```python
from build123d import *

# Parameters (mm, degrees)
CROQUIS1_W                      = 64
CROQUIS1_H                      = 120
CROQUIS1_R                      = 1.5
CROQUIS1_W_2                    = 2
CROQUIS1_H_2                    = 40
SALIENTE_EXTRUIR1_DEPTH         = 1
PLIEGUE_START                   = 63.746512
PLIEGUE_CROQUIZADO1_OUTLINE_W   = 120
PLIEGUE_CROQUIZADO1_OUTLINE_H   = 1
PLIEGUE_CROQUIZADO1_DEPTH       = 9.933488
PLIEGUE_START_2                 = 62.786512
PLIEGUE_CROQUIZADO1_2_OUTLINE_R = 1.5
PLIEGUE_CROQUIZADO1_2_DEPTH     = 1.213488
PLIEGUE_START_3                 = -121
PLIEGUE_CROQUIZADO1_3_DEPTH     = 122
PLIEGUE_START_4                 = -120
PLIEGUE_CROQUIZADO1_4_DEPTH     = 120
CORTAR_EXTRUIR1_REACH           = 138.485
CORTAR_EXTRUIR2_DEPTH           = 184
REDONDEO1_R                     = 4


with BuildPart() as part:
    # Croquis1 → Saliente-Extruir1 (new body)
    # profile 1 of 5: a face of its own
    with BuildSketch(Plane(origin=(0, 0, 0), x_dir=(0, 1, 0), z_dir=(0, 0, 1))):
        with Locations((32, 60)):
            Rectangle(CROQUIS1_W, CROQUIS1_H)
    # profile 2 of 5: a face of its own
    with BuildSketch(Plane(origin=(0, 0, 0), x_dir=(0, 1, 0), z_dir=(0, 0, 1))):
        Polygon((64, 120), (64, 0), (67.68, 0), (67.68, 25), (67.68, 40), (67.68, 80), (67.68, 95), (67.68, 120), align=None)
    # profile 3 of 5: a face of its own
    with BuildSketch(Plane(origin=(0, 0, 0), x_dir=(0, 1, 0), z_dir=(0, 0, 1))):
        Polygon((67.68, 40), (67.68, 25), (73.68, 25), (73.68, 40), (69.68, 40), align=None)
        with Locations(Location((69.68, 30, 0), (0, 0, 270))):
            Circle(CROQUIS1_R, mode=Mode.SUBTRACT)
    # profile 4 of 5: a face of its own
    with BuildSketch(Plane(origin=(0, 0, 0), x_dir=(0, 1, 0), z_dir=(0, 0, 1))):
        Polygon((73.68, 95), (67.68, 95), (67.68, 80), (69.68, 80), (73.68, 80), align=None)
        with Locations(Location((69.68, 90, 0), (0, 0, 270))):
            Circle(CROQUIS1_R, mode=Mode.SUBTRACT)
    # profile 5 of 5: a face of its own
    with BuildSketch(Plane(origin=(0, 0, 0), x_dir=(0, 1, 0), z_dir=(0, 0, 1))):
        with Locations((68.68, 60)):
            Rectangle(CROQUIS1_W_2, CROQUIS1_H_2)
    extrude(amount=SALIENTE_EXTRUIR1_DEPTH)

    # Pliegue croquizado1: read off the stored shape, not the designer's step
    # Pliegue croquizado1 outline → Pliegue croquizado1 (cut)
    with BuildSketch(Plane(origin=(0, 0, 0), x_dir=(1, 0, 0), z_dir=(0, 1, 0)).offset(PLIEGUE_START)):
        with Locations((-60, -0.5)):
            Rectangle(PLIEGUE_CROQUIZADO1_OUTLINE_W, PLIEGUE_CROQUIZADO1_OUTLINE_H)
    extrude(amount=PLIEGUE_CROQUIZADO1_DEPTH, mode=Mode.SUBTRACT)

    # Pliegue croquizado1 2 outline → Pliegue croquizado1 2 (add)
    with BuildSketch(Plane(origin=(0, 0, 0), x_dir=(1, 0, 0), z_dir=(0, 1, 0)).offset(PLIEGUE_START_2)):
        Polygon((-95, -11.495486979), (-80, -11.495486979), (-80, -7.495486979), (-40, -7.495486979), (-40, -11.495486979), (-25, -11.495486979), (-25, -5.495486979), (0, -5.495486979), (0, -1), (-120, -1), (-120, -5.495486979), (-95, -5.495486979), align=None)
        with Locations((-90, -7.495486979)):
            Circle(PLIEGUE_CROQUIZADO1_2_OUTLINE_R, mode=Mode.SUBTRACT)
        with Locations((-30, -7.495486979)):
            Circle(PLIEGUE_CROQUIZADO1_2_OUTLINE_R, mode=Mode.SUBTRACT)
    extrude(amount=PLIEGUE_CROQUIZADO1_2_DEPTH)

    # Pliegue croquizado1 3 outline → Pliegue croquizado1 3 (cut)
    with BuildSketch(Plane.YZ.offset(PLIEGUE_START_3)):
        with BuildLine():
            Line((63, 11.495486979), (62.786512, 11.495486979))
            Line((62.786512, 11.495486979), (62.786512, 1.656905608))
            ThreePointArc((62.786512, 1.656905608), (62.945569917, 2.013423228), (63, 2.4))
            Line((63, 2.4), (63, 11.495486979))
        make_face()
        with BuildLine():
            Line((64, 1), (64, 2.4))
            ThreePointArc((64, 2.4), (63.297056275, 0.702943725), (61.6, 0))
            Line((61.6, 0), (63.746512, 0))
            Line((63.746512, 0), (63.746512, 1))
            Line((63.746512, 1), (64, 1))
        make_face()
    extrude(amount=PLIEGUE_CROQUIZADO1_3_DEPTH, mode=Mode.SUBTRACT)

    # Pliegue croquizado1 4 outline → Pliegue croquizado1 4 (add)
    with BuildSketch(Plane.YZ.offset(PLIEGUE_START_4)):
        with BuildLine():
            Line((62.786512, 1), (62.786512, 1.656905608))
            ThreePointArc((62.786512, 1.656905608), (62.278110556, 1.175187331), (61.6, 1))
            Line((61.6, 1), (62.786512, 1))
        make_face()
    extrude(amount=PLIEGUE_CROQUIZADO1_4_DEPTH)

    # Simetría1: part across plane


with BuildPart() as part_1:
    add(part.part)
    add(part.part.mirror(Plane(origin=(0, 0, 1), x_dir=(0, 0, 1), z_dir=(0, 1, 0))))

    # Croquis7 → Cortar-Extruir1 (cut, up to next)
    with BuildSketch(Plane(origin=(0, 0, 0), x_dir=(-1, 0, 0), z_dir=(0, 0, -1)), mode=Mode.PRIVATE) as cortar_extruir1_sk1:
        with BuildLine():
            Line((35, 45.000000776), (35, -45.000000776))
            ThreePointArc((35, -45.000000776), (40.000000388, -50), (45, -45))
            Line((45, -45), (45, 45))
            ThreePointArc((45, 45), (40.000000388, 50), (35, 45.000000776))
        make_face()
    cortar_extruir1_tool1 = extrude(cortar_extruir1_sk1.sketch, amount=-CORTAR_EXTRUIR1_REACH, mode=Mode.PRIVATE) & part_1.part
    # Croquis7 → Cortar-Extruir1 (cut, up to next)
    with BuildSketch(Plane(origin=(0, 0, 0), x_dir=(-1, 0, 0), z_dir=(0, 0, -1)), mode=Mode.PRIVATE) as cortar_extruir1_sk2:
        with BuildLine():
            Line((15, 45.000000776), (15, -45.000000776))
            ThreePointArc((15, -45.000000776), (20.000000388, -50), (25, -45))
            Line((25, -45), (25, 45))
            ThreePointArc((25, 45), (20.000000388, 50), (15, 45.000000776))
        make_face()
    cortar_extruir1_tool2 = extrude(cortar_extruir1_sk2.sketch, amount=-CORTAR_EXTRUIR1_REACH, mode=Mode.PRIVATE) & part_1.part
    # Croquis7 → Cortar-Extruir1 (cut, up to next)
    with BuildSketch(Plane(origin=(0, 0, 0), x_dir=(-1, 0, 0), z_dir=(0, 0, -1)), mode=Mode.PRIVATE) as cortar_extruir1_sk3:
        with BuildLine():
            Line((55, 45.000000776), (55, -45.000000776))
            ThreePointArc((55, -45.000000776), (60.000000388, -50), (65, -45))
            Line((65, -45), (65, 45))
            ThreePointArc((65, 45), (60.000000388, 50), (55, 45.000000776))
        make_face()
    cortar_extruir1_tool3 = extrude(cortar_extruir1_sk3.sketch, amount=-CORTAR_EXTRUIR1_REACH, mode=Mode.PRIVATE) & part_1.part
    # Croquis7 → Cortar-Extruir1 (cut, up to next)
    with BuildSketch(Plane(origin=(0, 0, 0), x_dir=(-1, 0, 0), z_dir=(0, 0, -1)), mode=Mode.PRIVATE) as cortar_extruir1_sk4:
        with BuildLine():
            Line((75, 45.000000776), (75, -45.000000776))
            ThreePointArc((75, -45.000000776), (80.000000388, -50), (85, -45))
            Line((85, -45), (85, 45))
            ThreePointArc((85, 45), (80.000000388, 50), (75, 45.000000776))
        make_face()
    cortar_extruir1_tool4 = extrude(cortar_extruir1_sk4.sketch, amount=-CORTAR_EXTRUIR1_REACH, mode=Mode.PRIVATE) & part_1.part
    # Croquis7 → Cortar-Extruir1 (cut, up to next)
    with BuildSketch(Plane(origin=(0, 0, 0), x_dir=(-1, 0, 0), z_dir=(0, 0, -1)), mode=Mode.PRIVATE) as cortar_extruir1_sk5:
        with BuildLine():
            Line((95, 45.000000776), (95, -45.000000776))
            ThreePointArc((95, -45.000000776), (100.000000388, -50), (105, -45))
            Line((105, -45), (105, 45))
            ThreePointArc((105, 45), (100.000000388, 50), (95, 45.000000776))
        make_face()
    cortar_extruir1_tool5 = extrude(cortar_extruir1_sk5.sketch, amount=-CORTAR_EXTRUIR1_REACH, mode=Mode.PRIVATE) & part_1.part
    add(cortar_extruir1_tool1.solids().sort_by_distance((-40, 0, 0))[0], mode=Mode.SUBTRACT)
    add(cortar_extruir1_tool2.solids().sort_by_distance((-20, 0, 0))[0], mode=Mode.SUBTRACT)
    add(cortar_extruir1_tool3.solids().sort_by_distance((-60, 0, 0))[0], mode=Mode.SUBTRACT)
    add(cortar_extruir1_tool4.solids().sort_by_distance((-80, 0, 0))[0], mode=Mode.SUBTRACT)
    add(cortar_extruir1_tool5.solids().sort_by_distance((-100, 0, 0))[0], mode=Mode.SUBTRACT)

    # Croquis8 → Cortar-Extruir2 (cut)
    with BuildSketch(Plane.XZ.offset(64)):
        Polygon((-80, 11.495486979), (-85, 11.495486979), (-85, 5.495486979), (-80, 5.495486979), (-40, 5.495486979), (-35, 5.495486979), (-35, 11.495486979), (-40, 11.495486979), (-40, 7.495486979), (-80, 7.495486979), align=None)
    extrude(amount=-CORTAR_EXTRUIR2_DEPTH, mode=Mode.SUBTRACT)

    # Redondeo1
    redondeo1_edges = [part_1.edges().sort_by_distance(p)[0] for p in [
        (-95, -63.5, 11.495486979),
        (-25, -63.5, 11.495486979),
        (-25, 63.5, 11.495486979),
        (-95, 63.5, 11.495486979),
        (-35, 63.5, 11.495486979),
        (-85, 63.5, 11.495486979),
        (-35, -63.5, 11.495486979),
        (-85, -63.5, 11.495486979),
    ]]
    fillet(redondeo1_edges, radius=REDONDEO1_R)


solid = part_1.part
```
Geometry check sheet. Reference: the model listing, model coordinates, mm. A direction names the side the tool comes from. Coordinates: 2 decimals unless noted, no trailing zeros. Loops run counter-clockwise (first coordinate to the right, second up) from the corner with the lowest first, then second, coordinate; pieces in that order, holes last. Notation, with made-up numbers: (81, 66) - (118, 66) arc R32 ccw to (118, 92) - close; hole circle Ø3 at (80.25, -14.5). An arc over 180 degrees is marked (long way). One line per item, written item: value. Start each with the question number.
(1) Cross-section at B-B on y = 15. Enter the section's corners in (x, z), plus the area to 3 significant figures.
(2) Tool access check on faces 5 (the cylindrical face through (-19.9, -50, 0.5)), 6 (the flat face through (-61, -63, 5)), 7 (the cylindrical face through (-33.86, -63.49, 10.29)). Record the directions out of +Z, -Z, +X, -X, +Y, -Y that give a thin tool (end or side, any length) a straight path to the whole face; none if there is none.
(3) Depth check by flat-ended pin: P1, Ø5, axis at x = -79, z = 9.5, coming from the -Y side; P2, Ø1.1, axis at x = -108, y = 63.5, coming from the +Z side; P3, Ø0.5, axis at y = 63.5, z = 6, coming from the -X side. Enter the tip coordinate at first touch or a pass-through.
(4) Mould release check, pull along Y, two halves, no side actions. Record for faces 1 (the cylindrical face through (-88.57, 63.49, 7.04)), 2 (the cylindrical face through (-20.1, 50, 0.5)), 3 (the flat face through (-61, -64, 5)), 4 (the cylindrical face through (-100.1, 50, 0.5)): released by +Y, released by -Y, zero draft, split by the parting line, or undercut.
(5) Material ranges on line 1 (Y direction, x = -89, z = 4.25); line 2 (Z direction, x = -97.5, y = -52); line 3 (Y direction, x = -5, z = 2), recorded low to high. Write a range as [from, to].
(6) Cross-section at A-A on x = -97. Enter the section's corners in (y, z), plus the area to 3 significant figures.
(7) Cross-section at C-C on y = 54. Enter the section's corners in (x, z).
Results below:
1. outline: (-120, 0) - (-105, 0) - (-105, 1) - (-120, 1) - close; (-95, 0) - (-85, 0) - (-85, 1) - (-95, 1) - close; (-75, 0) - (-65, 0) - (-65, 1) - (-75, 1) - close; (-55, 0) - (-45, 0) - (-45, 1) - (-55, 1) - close; (-35, 0) - (-25, 0) - (-25, 1) - (-35, 1) - close; (-15, 0) - (0, 0) - (0, 1) - (-15, 1) - close
1. area: 70.0 mm2
2. face 5: +Z, -Z
2. face 6: +Z, +X, -X
2. face 7: +Z, +Y, -Y
3. P1: passes through
3. P2: stops at z = 5.5
3. P3: stops at x = -95
4. face 1: zero draft
4. face 2: undercut
4. face 3: released by -Y
4. face 4: undercut
5. line 1: y = [-64, -63], [63, 64]
5. line 2: z = [0, 1]
5. line 3: y = [-63.97, -62.94], [62.94, 63.97]
6. outline: (-64, 2.4) arc R2.4 ccw to (-61.6, 0) - (-49, 0) - (-49, 1) - (-61.6, 1) arc R1.4 cw to (-63, 2.4) - (-63, 5.5) - (-64, 5.5) - close; (49, 0) - (61.6, 0) arc R2.4 ccw to (64, 2.4) - (64, 5.5) - (63, 5.5) - (63, 2.4) arc R1.4 cw to (61.6, 1) - (49, 1) - close
6. area: 37.4 mm2
7. outline: (-120, 0) - (0, 0) - (0, 1) - (-120, 1) - close
